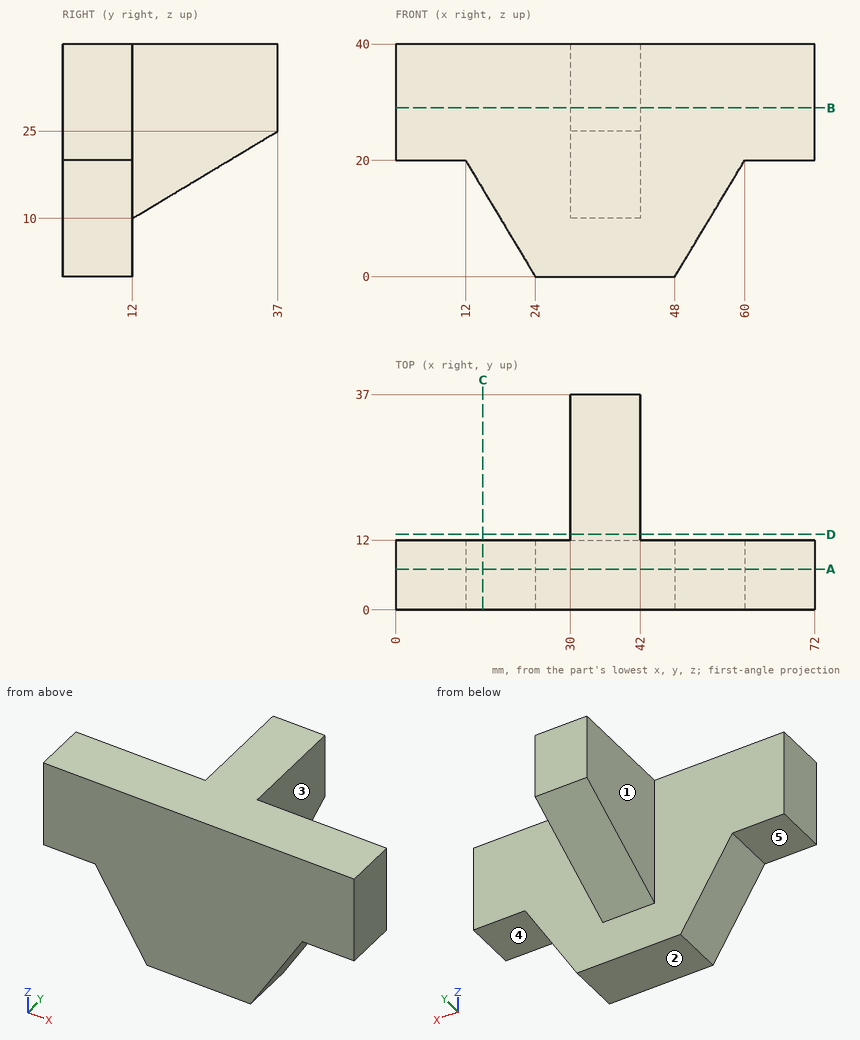
Check sheet for the drawn part. Datum: minimum x, y, z corner. Units: mm. A direction names the side the tool comes from. Give positions to 0.01 mm unless a question says otherwise; leave off trailing zeros. Order: outer loops, then holes, each group sorted by start corner. A loop starts at its lowest first (then second) coordinate and runs counter-clockwise, first axis right, second up. Notation, with made-up numbers: (-12.5, 34) -> (11.5, 34) arc R16 cw to (11.5, 41) -> close; hole circle Ø1 at (72, -7). An arc over 180 degrees is marked (long way). Use a Markdown table: item, result.
1) Section check A-A, the plane y = 7. Record the boundary of the cut face in (x, z), then the cut area to 3 significant figures.
Results:
| item | result |
|---|---|
| outline | (0, 20) -> (12, 20) -> (24, 0) -> (48, 0) -> (60, 20) -> (72, 20) -> (72, 40) -> (0, 40) -> close |
| area | 2,160 mm² |
2) Tool access check on the marked faces 1, 2, 3, 4 and 5. Record the directions out of +Z, -Z, +X, -X, +Y, -Y that give a thin tool (end or side, any length) a straight path to the whole face; none if there is none.
Results:
| item | result |
|---|---|
| face 1 | +Z, -Z, -X, +Y |
| face 2 | -Z, +X, -X, +Y, -Y |
| face 3 | +Z, -Z, +X, +Y |
| face 4 | -Z, +X, +Y, -Y |
| face 5 | -Z, -X, +Y, -Y |
3) Depth check by flat-ended pin: pin 1 Ø5 at (x, y) = (64, 8) entering from -Z; pin 2 Ø5 at (y, z) = (23.5, 29) entering from +X; pin 3 Ø20 at (y, z) = (25.5, 27) entering from -X. Enter the tip coordinate at first touch or a pass-through.
Results:
| item | result |
|---|---|
| pin 1 | z = 20 |
| pin 2 | x = 42 |
| pin 3 | x = 30 |
4) Section check D-D, the plane y = 13. Record the boundary of the cut face in (x, z).
Results:
| item | result |
|---|---|
| outline | (30, 10.6) -> (42, 10.6) -> (42, 40) -> (30, 40) -> close |
5) Section check B-B, the plane z = 29. Record the boundary of the cut face in (x, y), then the cut area to 3 significant figures.
Results:
| item | result |
|---|---|
| outline | (0, 0) -> (72, 0) -> (72, 12) -> (42, 12) -> (42, 37) -> (30, 37) -> (30, 12) -> (0, 12) -> close |
| area | 1,160 mm² |
6) Section check C-C, the plane x = 15. Record the boundary of the cut face in (y, z), then the cut area to 3 significant figures.
Results:
| item | result |
|---|---|
| outline | (0, 15) -> (12, 15) -> (12, 40) -> (0, 40) -> close |
| area | 300 mm² |
7) Material ranges on probe 1 along Y at (x, z) = (26, 2.5); probe 2 along X at (y, z) = (20, 25.5); probe 3 along Z at (x, y) = (69, 7), recorded low to high.
Results:
| item | result |
|---|---|
| probe 1 | 0 to 12 |
| probe 2 | 30 to 42 |
| probe 3 | 20 to 40 |
